Autodesk Inventor part; units mm, degrees
ref_plane "YZ Plane" through (0, 0, 0) normal (1, 0, 0) x (0, 1, 0)
ref_plane "XZ Plane" through (0, 0, 0) normal (0, 1, 0) x (-1, 0, 0)
ref_plane "XY Plane" through (0, 0, 0) normal (0, 0, 1) x (1, 0, 0)
sketch "Sketch1" plane through (0, 0, 0) normal (0, 1, 0) x (-1, 0, 0)
  line L0 (40, 20) -> (-40, 20)
  line L1 (-40, 20) -> (-40, -20)
  line L2 (-40, -20) -> (40, -20)
  line L3 (40, -20) -> (40, 20)
  line L4 (40, 20) -> (-40, -20) construction
  line L5 (-40, 20) -> (40, -20) construction
  point P0 (0, 0)
  dimension "d0" = 80
  dimension "d1" = 40
extrude "Extrusion1" add sketch "Sketch1" along normal blind 8
shell "Shell1" thickness 1.6 removed faces 1 at (13.3333, 0, 6.6667)
fillet "Fillet1" radius 0.5 20 edges at (0, 8, 20) (-40, 8, 0) (-40, 4, 20) (-40, 0, 0) (0, 0, 20) (40, 4, 20) (-40, 4, -20) (0, 0, -20) (0, 8, -20) (40, 4, -20) (40, 8, 0) (38.4, 0, 0) (40, 0, 0) (0, 0, 18.4) (0, 0, -18.4) (-38.4, 0, 0) (38.4, 6.4, 0) (0, 6.4, -18.4) (0, 6.4, 18.4) (-38.4, 6.4, 0)
sketch "Sketch4" plane through (-37.9, 6.4, 17.9) normal (0, -1, 0) x (1, 0, 0)
  circle A0 centre (36.9, -25.855) radius 1.5
  circle A1 centre (24, -25.855) radius 1.5
  circle A2 centre (24, -9.945) radius 1.5
  circle A3 centre (36.9, -9.945) radius 1.5
  line L0 (0, -35.8) -> (0, 0)
  line L1 (0, -17.9) -> (71.9831, -17.9)
  line L2 (36.9, -9.945) -> (24, -25.855) construction
  line L3 (24, -9.945) -> (36.9, -25.855) construction
  line L4 (40.9, -5.945) -> (20, -5.945)
  line L5 (20, -5.945) -> (20, -29.855)
  line L6 (20, -29.855) -> (40.9, -29.855)
  line L7 (40.9, -29.855) -> (40.9, -5.945)
  line L8 (40.9, -5.945) -> (20, -29.855) construction
  line L9 (20, -5.945) -> (40.9, -29.855) construction
  point P0 (30.45, -17.9)
  dimension "d24" = 3
  dimension "d25" = 3
  dimension "d28" = 15.91
  dimension "d29" = 12.9
  dimension "d30" = 4
  dimension "d31" = 4
  dimension "d32" = 20
extrude "Extrusion4" add sketch "Sketch4" along normal blind 4
equation "\"d0\" = plate_depth"
equation "\"d1\" = plate_width"
equation "\"plate_width\" = 40"
equation "\"plate_depth\" = 80"
properties part number "plate"
Build history of the part. All positions in model axes, mm. A direction names the side the tool comes from. Round coordinates to 2 decimals unless told otherwise and drop trailing zeros. Write each loop counter-clockwise with the first axis right and the second up, starting at its lowest first coordinate (ties: lowest second). Pieces come first, ordered by that corner, then holes. Notation, with made-up numbers: (25.25, -3.5) - (38.25, -3.5) arc R19 cw to (38.25, 13.5) - close; hole circle Ø4 at (34, -16.75). An arc over 180 degrees is marked (long way). Answer as CSV lines item,"result".
Q1. Cut at C-C (y = 1.25). Write the cut outline in (x, z).
Report:
outline,"(-40, -19.5) arc R0.5 ccw to (-39.5, -20) - (39.5, -20) arc R0.5 ccw to (40, -19.5) - (40, 19.5) arc R0.5 ccw to (39.5, 20) - (-39.5, 20) arc R0.5 ccw to (-40, 19.5) - close; hole (-38.4, -18.4) - (38.4, -18.4) - (38.4, 18.4) - (-38.4, 18.4) - close"
Q2. Drill centre lines: probe 1 along X at (y, z) = (3.5, -6); probe 2 along Z at (x, y) = (-13.9, 5.5) (3 decimals); probe 3 along Z at (x, y) = (-4, 4.5) (3 decimals). Where is each one in solid material? Low to high. Write a range as [from, to].
Report:
probe 1,"x = [-40, -38.4], [-17.9, 3], [38.4, 40]"
probe 2,"z = [-20, -18.4], [-11.955, -9.455], [-6.455, 6.455], [9.455, 11.955], [18.4, 20]"
probe 3,"z = [-20, -18.4], [-11.955, 11.955], [18.4, 20]"
Q3. Cut at B-B (x = -25.5). Write the cut outline in (y, z), and give its area (3 significant figures).
Report:
outline,"(0, -19.5) arc R0.5 ccw to (0.5, -20) - (7.5, -20) arc R0.5 ccw to (8, -19.5) - (8, 19.5) arc R0.5 ccw to (7.5, 20) - (0.5, 20) arc R0.5 ccw to (0, 19.5) - (0, 18.9) arc R0.5 ccw to (0.5, 18.4) - (5.9, 18.4) arc R0.5 cw to (6.4, 17.9) - (6.4, -17.9) arc R0.5 cw to (5.9, -18.4) - (0.5, -18.4) arc R0.5 ccw to (0, -18.9) - close"
area,"84.3 mm^2"
Q4. Pull direction Z, two halves, no side cores. Call faces 3 (the cylindrical face through (-2.19, 4.43, 8.87)), 4 (the flat face through (1, 4, -20)), 5 (the flat face through (40, 4, 0)): +Z half, -Z half, draft (parallel to the pull), parting line (faces both ways), or undercut.
Report:
face 3,"undercut"
face 4,"-Z half"
face 5,"draft"
Q5. Cut at A-A (y = 4.5). Write the cut outline in (x, z) (3 decimals).
Report:
outline,"(-40, -19.5) arc R0.5 ccw to (-39.5, -20) - (39.5, -20) arc R0.5 ccw to (40, -19.5) - (40, 19.5) arc R0.5 ccw to (39.5, 20) - (-39.5, 20) arc R0.5 ccw to (-40, 19.5) - close; (-17.9, -11.955) - (3, -11.955) - (3, 11.955) - (-17.9, 11.955) - close; hole (-38.4, -18.4) - (38.4, -18.4) - (38.4, 18.4) - (-38.4, 18.4) - close; hole circle Ø3 at (-13.9, -7.955); hole circle Ø3 at (-13.9, 7.955); hole circle Ø3 at (-1, -7.955); hole circle Ø3 at (-1, 7.955)"
Q6. Cut at D-D (z = -1). Write the cut outline in (x, y), and give its area (3 significant figures).
Report:
outline,"(-40, 0.5) arc R0.5 ccw to (-39.5, 0) - (-38.9, 0) arc R0.5 ccw to (-38.4, 0.5) - (-38.4, 5.9) arc R0.5 cw to (-37.9, 6.4) - (-17.9, 6.4) - (-17.9, 2.4) - (3, 2.4) - (3, 6.4) - (37.9, 6.4) arc R0.5 cw to (38.4, 5.9) - (38.4, 0.5) arc R0.5 ccw to (38.9, 0) - (39.5, 0) arc R0.5 ccw to (40, 0.5) - (40, 7.5) arc R0.5 ccw to (39.5, 8) - (-39.5, 8) arc R0.5 ccw to (-40, 7.5) - close"
area,"232 mm^2"
Q7. Tool access for faces 1 (the flat face through (-1, 6.4, -8)), 2 (the flat face through (1, 8, 0)): list every direction of +Z, -Z, +X, -X, +Y, -Y with a clear straight run to the whole face (end or side of a thin tool).
Report:
face 1,"-Y"
face 2,"+Z, -Z, +X, -X, +Y"
Q8. Drop flat-ended pins along their axis: pin 1 (6.5 mm diameter, centred on x = -9, z = 3, fed in from -Y); pin 2 (2.5 mm diameter, centred on x = -13.9, z = 7.955, fed in from -Y). Give the stop position or say it passes through.
Report:
pin 1,"stops at y = 2.4"
pin 2,"stops at y = 6.4"
